The drawing under review shows one solid part. Ordinate dimensions are in mm from its lowest x, y, z. A direction names the side the tool comes from. Round coordinates to 2 decimals unless told otherwise and drop trailing zeros. Loops run counter-clockwise (first coordinate to the right, second up) from the corner with the lowest first, then second, coordinate; pieces in that order, holes last. Notation, with made-up numbers: (38, 36.5) -> (84, 36.5) arc R13 cw to (84, 41.5) -> close; hole circle Ø10 at (-12, -26.5). An arc over 180 degrees is marked (long way). Use a Markdown table: item, result. Add a question column.
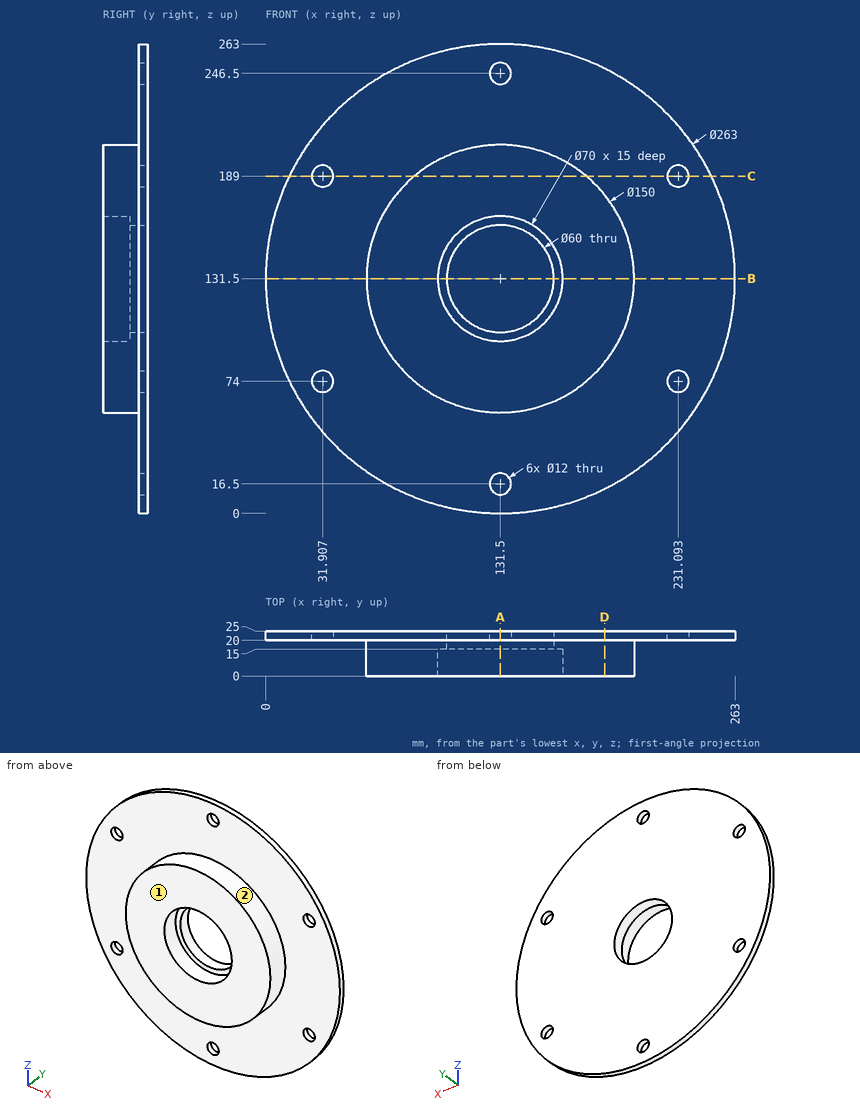
1. Consider section B-B on z = 131.5. State the section outline as (x, y) points.
2. For the marked faces 1 and 2, list the 3-axis set-ups (+Z, -Z, +X, -X, +Y, -Y) from which the entire face can be reached by the end or side of a thin tool; tool diameter is ignored.
3. Consider section C-C on z = 189. State the section outline as (x, y) points.
4. Consider section D-D on x = 190. State the section outline as (y, z) points, plus the area to 4 significant figures.
5. Consider section A-A on x = 131.5. State the section outline as (y, z) points.
6. To check wall thickness, follow probe 1 along Z at (x, y) = (131.5, 23); probe 2 along Z at (x, y) = (37, 20.5); probe 3 along X at (y, z) = (19.75, 132). State the ranges of each line that lie inside material, in increasing order. Write a range as from..to.
7. Insertion check: P1, Ø15.5, axis at x = 131.5, z = 16.5, coming from the -Y side; P2, Ø8, axis at x = 27, y = 13, coming from the -Z side; P3, Ø1, axis at x = 152.5, y = 8, coming from the -Z side; P4, Ø8, axis at x = 176.5, y = 13.5, coming from the -Z side. Each pin has a flat end and moves straight along its axis. Give the tip position at first contact, or say it passes through.
Verdict:
| question | item | result |
|---|---|---|
| 1 | outline | (0, 20) -> (56.5, 20) -> (56.5, 0) -> (96.5, 0) -> (96.5, 15) -> (101.5, 15) -> (101.5, 25) -> (0, 25) -> close; (161.5, 15) -> (166.5, 15) -> (166.5, 0) -> (206.5, 0) -> (206.5, 20) -> (263, 20) -> (263, 25) -> (161.5, 25) -> close |
| 2 | face 1 | +Z, -Z, +X, -X, -Y |
| 2 | face 2 | -Y |
| 3 | outline | (13.24, 20) -> (25.91, 20) -> (25.91, 25) -> (13.24, 25) -> close; (37.91, 20) -> (83.35, 20) -> (83.35, 0) -> (179.65, 0) -> (179.65, 20) -> (225.09, 20) -> (225.09, 25) -> (37.91, 25) -> close; (237.09, 20) -> (249.76, 20) -> (249.76, 25) -> (237.09, 25) -> close |
| 4 | outline | (0, 84.57) -> (20, 84.57) -> (20, 13.73) -> (25, 13.73) -> (25, 249.27) -> (20, 249.27) -> (20, 178.43) -> (0, 178.43) -> close |
| 4 | area | 3,055 mm² |
| 5 | outline | (0, 56.5) -> (20, 56.5) -> (20, 22.5) -> (25, 22.5) -> (25, 101.5) -> (15, 101.5) -> (15, 96.5) -> (0, 96.5) -> close; (0, 166.5) -> (15, 166.5) -> (15, 161.5) -> (25, 161.5) -> (25, 240.5) -> (20, 240.5) -> (20, 206.5) -> (0, 206.5) -> close; (20, 0) -> (25, 0) -> (25, 10.5) -> (20, 10.5) -> close; (20, 252.5) -> (25, 252.5) -> (25, 263) -> (20, 263) -> close |
| 6 | probe 1 | z = 0..10.5, 22.5..101.5, 161.5..240.5, 252.5..263 |
| 6 | probe 2 | z = 40.06..70.83, 77.17..185.83, 192.17..222.94 |
| 6 | probe 3 | x = 56.5..101.5, 161.5..206.5 |
| 7 | P1 | stops at y = 20 |
| 7 | P2 | passes through |
| 7 | P3 | stops at z = 59.36 |
| 7 | P4 | stops at z = 68.7 |
